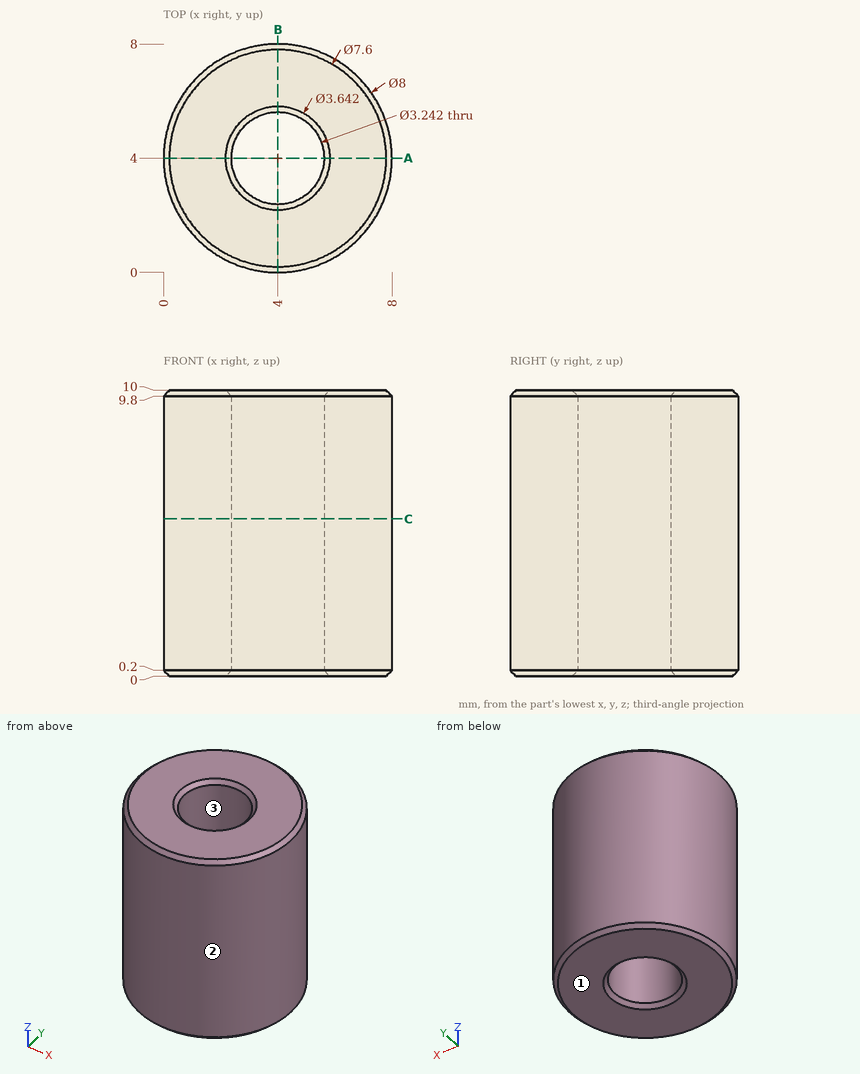
Job drawing, mm, ordinate dimensions from the low corner. One solid piece. Coordinates: 2 decimals unless noted, no trailing zeros. Order: outer loops, then holes, each group sorted by start corner. A loop starts at its lowest first (then second) coordinate and runs counter-clockwise, first axis right, second up. Notation, with made-up numbers: (5, 83) - (59, 83) arc R11 ccw to (59, 94) - close; hole circle Ø8 at (41, 72). An arc over 180 degrees is marked (long way). Return JSON: item names as keys, results as strings. Group by question number.
1) Mould opens along Y. For the marked faces 1, 2 and 3 say: released by +Y, released by -Y, zero draft, split by the parting line, or undercut.
2) Probe line 1 (Y direction, x = 4, z = 5.25); line 2 (Y direction, x = 5, z = 2); line 3 (X direction, y = 0.75, z = 4.5). List the from-to ranges inside material, lowest first. Write a range as from..to.
3) Saw through at A-A, the plane y = 4. Write the cut outline in (x, z).
4) Flat gauge pin, fed straight in: P1, Ø3, axis at x = 4, y = 4, coming from the -Z side. Where does the tip first touch, or does it go through?
5) Saw through at C-C, the plane z = 5.5. Write the cut outline in (x, y), plus the area to 3 significant figures.
Values found:
{
 "1": {"face 1": "zero draft", "face 2": "split by the parting line", "face 3": "undercut"},
 "2": {"line 1": "y = 0..2.38, 5.62..8", "line 2": "y = 0.13..2.72, 5.28..7.87", "line 3": "x = 1.67..6.33"},
 "3": {"outline": "(0, 0.2) - (0.2, 0) - (2.18, 0) - (2.38, 0.2) - (2.38, 9.8) - (2.18, 10) - (0.2, 10) - (0, 9.8) - close; (5.62, 0.2) - (5.82, 0) - (7.8, 0) - (8, 0.2) - (8, 9.8) - (7.8, 10) - (5.82, 10) - (5.62, 9.8) - close"},
 "4": {"P1": "passes through"},
 "5": {"outline": "circle Ø8 at (4, 4); hole circle Ø3.24 at (4, 4)", "area": "42.0 mm²"}
}
